Design review of the part built by this model. Coordinates are the model's own, in mm. A direction names the side the tool comes from. Round coordinates to 2 decimals unless told otherwise and drop trailing zeros. Loops run counter-clockwise (first coordinate to the right, second up) from the corner with the lowest first, then second, coordinate; pieces in that order, holes last. Notation, with made-up numbers: M -26,36 L 26,36 A22 ccw 26,74 Z; hole C 38,85.25 d11. An arc over 180 degrees is marked long. One line per item, written item: value. Start each with the question number.
Item 1: For faces 5 (the flat face through (12, 4, 10)), 6 (the cylindrical face through (1.699, 5.042, 19.715)), 7 (the flat face through (10, 5, 10)), 8 (the flat face through (7.5, 1, 10)), 9 (the cylindrical face through (1.699, 5.042, 0.285)), list the 3-axis set-ups (+Z, -Z, +X, -X, +Y, -Y) from which the entire face can be reached by the end or side of a thin tool; tool diameter is ignored.
Item 2: Clearance check with flat-ended pins moving along their axes: pin 1 (1.5 mm diameter, centred on x = 8, y = 5, fed in from +Z); pin 2 (5 mm diameter, centred on x = 6, z = 9, fed in from +Y). State where each tip first meets the part, or that it passes through.
Item 3: For line 1 along X through (y, z) = (0.5, 14.5); line 2 along X through (y, z) = (5.5, 18.25); line 3 along Y through (x, z) = (3.25, 2.75), list the stretches that pass through material, from the lowest coordinate up.
Item 4: We need section C-C (z = 11). Write out the cut boundary in (x, y).
Item 5: We need section A-A (x = 6). Write out the cut boundary in (y, z), then the cut area to 3 significant figures.
Item 6: We need section D-D (y = 0.75). Write out the cut boundary in (x, z), then the cut area to 3 significant figures.
Item 7: Mouldability with a two-part tool opening along Z and no side actions: class faces 1 (the flat face through (6, 1, 20)), 2 (the flat face through (4.5, 1, 10)), 3 (the flat face through (11, 8, 10)), 4 (the cylindrical face through (10.301, 4.958, 0.285)) as released by +Z, released by -Z, zero draft, split by the parting line, or undercut.
Item 8: We need section B-B (y = 4). Write out the cut boundary in (x, z).
from build123d import *

# Parameters (mm, degrees)
EXTRUDE_DEPTH = 20
POCKET_DEPTH  = 5
FILLET_R      = 1
FILLET001_R   = 0.5


with BuildPart() as part:
    # Sketch → Extrude (new body)
    with BuildSketch(Plane.XY):
        Polygon((0, 0), (12, 0), (12, 8), (10, 8), (10, 2), (2, 2), (2, 8), (0, 8), align=None)
    extrude(amount=EXTRUDE_DEPTH)

    # Sketch001 (on Face5 of BaseFeature) → Pocket (cut)
    with BuildSketch(Plane(origin=(0, 2, 0), x_dir=(-1, 0, 0), z_dir=(0, 1, 0))):
        with BuildLine():
            ThreePointArc((-4.5, 15), (-6, 16.5), (-7.5, 15))
            Line((-7.5, 15), (-7.5, 5))
            ThreePointArc((-7.5, 5), (-6, 3.5), (-4.5, 5))
            Line((-4.5, 15), (-4.5, 5))
        make_face()
    extrude(amount=-POCKET_DEPTH, mode=Mode.SUBTRACT)

    # Fillet
    fillet_edges = [part.edges().sort_by_distance(p)[0] for p in [
        (11, 8, 0),
        (10, 5, 0),
        (2, 5, 0),
        (1, 8, 0),
        (11, 8, 20),
        (10, 5, 20),
        (2, 5, 20),
        (1, 8, 20),
    ]]
    fillet(fillet_edges, radius=FILLET_R)

    # Fillet001
    fillet001_edges = [part.edges().sort_by_distance(p)[0] for p in [
        (0, 3.5, 0),
        (12, 3.5, 0),
    ]]
    fillet(fillet001_edges, radius=FILLET001_R)


solid = part.part
A:
1. face 5: +Z, -Z, +X, +Y, -Y
1. face 6: +Z, +Y
1. face 7: +Z, -Z, +Y
1. face 8: +Y, -Y
1. face 9: -Z, +Y
2. pin 1: through
2. pin 2: y = 2
3. line 1: 0 to 4.5, 7.5 to 12
3. line 2: 0 to 2, 10 to 12
3. line 3: 0 to 2
4. outline: M 0,0 L 4.5,0 L 4.5,2 L 2,2 L 2,8 L 0.5,8 A0.5 ccw 0,7.5 Z; M 7.5,0 L 12,0 L 12,7.5 A0.5 ccw 11.5,8 L 10,8 L 10,2 L 7.5,2 Z
5. outline: M 0,0 L 2,0 L 2,3.5 L 0,3.5 Z; M 0,16.5 L 2,16.5 L 2,20 L 0,20 Z
5. area: 14.0 mm2
6. outline: M 0,0.5 A0.5 ccw 0.5,0 L 11.5,0 A0.5 ccw 12,0.5 L 12,19.5 A0.5 ccw 11.5,20 L 0.5,20 A0.5 ccw 0,19.5 Z; hole M 4.5,5 A1.5 ccw 7.5,5 L 7.5,15 A1.5 ccw 4.5,15 Z
6. area: 203 mm2
7. face 1: released by +Z
7. face 2: undercut
7. face 3: zero draft
7. face 4: released by -Z
8. outline: M 0,0.5 A0.5 ccw 0.5,0 L 1,0 A1 ccw 2,1 L 2,19 A1 ccw 1,20 L 0.5,20 A0.5 ccw 0,19.5 Z; M 10,1 A1 ccw 11,0 L 11.5,0 A0.5 ccw 12,0.5 L 12,19.5 A0.5 ccw 11.5,20 L 11,20 A1 ccw 10,19 Z
